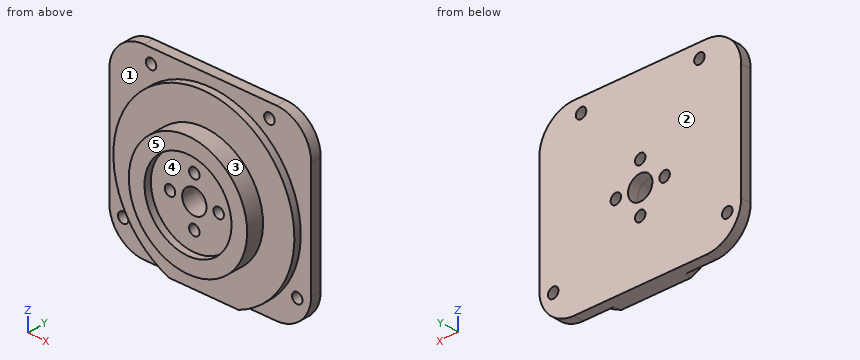
```python
from build123d import *
from build123d.topology import SkipClean

# Parameters (mm, degrees)
SKETCH_1_W          = 58
SKETCH_1_H          = 58
SKETCH_1_R          = 1.5
SKETCH_1_R_2        = 3.5
EXTRUDE_1_DEPTH     = 3
EXTRUDE_START       = 5
SKETCH_2_R          = 12.5
SKETCH_2_R_2        = 1.5
SKETCH_2_R_3        = 3.5
EXTRUDE_2_DEPTH     = 5
EXTRUDE_START_2     = 7
SKETCH_6_R          = 17
SKETCH_6_R_2        = 12.5
EXTRUDE_3_DEPTH     = 7
SKETCH_8_R          = 26
SKETCH_8_R_2        = 12
EXTRUDE_5_DEPTH     = 2
SKETCH_10_W         = 58
SKETCH_10_H         = 5
CUT_EXTRUDE_1_DEPTH = 10
FILLET_1_R          = 10


with BuildPart() as part:
    # 草图1 → 凸台-拉伸1 (new body)
    with BuildSketch(Plane(origin=(0, 0, 0), x_dir=(1, 0, 0), z_dir=(0, 1, 0))):
        Rectangle(SKETCH_1_W, SKETCH_1_H)
        with Locations(Location((0, 7, 0), (0, 0, 270))):
            Circle(SKETCH_1_R, mode=Mode.SUBTRACT)
        with Locations(Location((7, 0, 0), (0, 0, 270))):
            Circle(SKETCH_1_R, mode=Mode.SUBTRACT)
        with Locations(Location((0, 0, 0), (0, 0, 270))):
            Circle(SKETCH_1_R_2, mode=Mode.SUBTRACT)
        with Locations(Location((0, -7, 0), (0, 0, 90))):
            Circle(SKETCH_1_R, mode=Mode.SUBTRACT)
        with Locations(Location((-7, 0, 0), (0, 0, 90))):
            Circle(SKETCH_1_R, mode=Mode.SUBTRACT)
        with Locations(Location((25, 16, 0), (0, 0, 270))):
            Circle(SKETCH_1_R, mode=Mode.SUBTRACT)
        with Locations(Location((-25, 16, 0), (0, 0, 90))):
            Circle(SKETCH_1_R, mode=Mode.SUBTRACT)
        with Locations(Location((17, -25, 0), (0, 0, 270))):
            Circle(SKETCH_1_R, mode=Mode.SUBTRACT)
        with Locations(Location((-17, -25, 0), (0, 0, 90))):
            Circle(SKETCH_1_R, mode=Mode.SUBTRACT)
    extrude(amount=EXTRUDE_1_DEPTH)

    # 草图2 → 凸台-拉伸2 (add)
    with SkipClean():  # the faces are left unmerged after this step: merging them gives an invalid solid
        with BuildSketch(Plane.XZ.offset(EXTRUDE_START)):
            with Locations(Location((0, 0, 0), (0, 0, 270))):
                Circle(SKETCH_2_R)
            with Locations(Location((0, 7, 0), (0, 0, 270))):
                Circle(SKETCH_2_R_2, mode=Mode.SUBTRACT)
            with Locations(Location((0, 0, 0), (0, 0, 270))):
                Circle(SKETCH_2_R_3, mode=Mode.SUBTRACT)
            with Locations(Location((-7, 0, 0), (0, 0, 270))):
                Circle(SKETCH_2_R_2, mode=Mode.SUBTRACT)
            with Locations(Location((0, -7, 0), (0, 0, 270))):
                Circle(SKETCH_2_R_2, mode=Mode.SUBTRACT)
            with Locations(Location((7, 0, 0), (0, 0, 270))):
                Circle(SKETCH_2_R_2, mode=Mode.SUBTRACT)
        extrude(amount=-EXTRUDE_2_DEPTH)

    # 草图6 → 凸台-拉伸3 (add)
    with SkipClean():  # the faces are left unmerged after this step: merging them gives an invalid solid
        with BuildSketch(Plane.XZ.offset(EXTRUDE_START_2)):
            with Locations(Location((0, 0, 0), (0, 0, 270))):
                Circle(SKETCH_6_R)
            with Locations(Location((0, 0, 0), (0, 0, 270))):
                Circle(SKETCH_6_R_2, mode=Mode.SUBTRACT)
        extrude(amount=-EXTRUDE_3_DEPTH)

    # 草图8 → 凸台-拉伸5 (add)
    with SkipClean():  # the faces are left unmerged after this step: merging them gives an invalid solid
        with BuildSketch(Plane.XZ):
            with Locations(Location((0, 0, 0), (0, 0, 270))):
                Circle(SKETCH_8_R)
            Circle(SKETCH_8_R_2, mode=Mode.SUBTRACT)
        extrude(amount=EXTRUDE_5_DEPTH)

    # 草图10 → 切除-拉伸1 (cut)
    with BuildSketch(Plane(origin=(0, 3, 0), x_dir=(1, 0, 0), z_dir=(0, 1, 0))):
        with Locations((0, 26.5)):
            Rectangle(SKETCH_10_W, SKETCH_10_H)
    extrude(amount=-CUT_EXTRUDE_1_DEPTH, mode=Mode.SUBTRACT)

    # 圆角1
    fillet_1_edges = [part.edges().sort_by_distance(p)[0] for p in [
        (29, 1.5, 29),
        (-29, 1.5, 29),
        (29, 1.5, -24),
        (-29, 1.5, -24),
    ]]
    fillet(fillet_1_edges, radius=FILLET_1_R)


solid = part.part
```
For this review, take the finished solid that the model builds, in its own axes (mm). Face numbers are marked on the shaded views. A direction names the side the tool comes from. Give positions to 0.01 mm unless a question says otherwise; leave off trailing zeros. Write each loop counter-clockwise with the first axis right and the second up, starting at its lowest first coordinate (ties: lowest second). Pieces come first, ordered by that corner, then holes. Notation, with made-up numbers: M -3.75,26.5 L 3.25,26.5 A19 ccw 3.25,39.5 Z; hole C 71.25,14 d5. An arc over 180 degrees is marked long. Answer as a JSON object with one key per item and string values. Group by question number.
Item 1: Tool access review of the marked faces 1 and 2: name each direction out of +Z, -Z, +X, -X, +Y, -Y from which nothing blocks a thin tool from reaching the whole face with its end or side.
Item 2: For pin 1 Ø6 at (x, y) = (-21, 0) entering from -Z; pin 2 Ø1.8 at (x, z) = (17, 25) entering from +Y; pin 3 Ø8 at (x, z) = (-5, -1) entering from -Y; pin 4 Ø5 at (y, z) = (-3, -11) entering from +X, all flat-tipped, find the tip position at first contact; note any pin that passes through.
Item 3: Draft analysis for pull direction X (two halves, no side actions). For the marked faces 3, 4 and 5, state which applies: +X half, -X half, draft (parallel to the pull), parting line (faces both ways), or undercut.
Item 4: For probe 1 along X at (y, z) = (1.45, 0); probe 2 along Z at (x, y) = (0, 0.65); probe 3 along Z at (x, y) = (-17, 1.8), list the stretches that pass through material, from the lowest coordinate up. Write a range as [from, to].
Item 5: Consider section A-A on x = 0. Write out the cut boundary in (y, z).
Item 6: Consider section B-B on y = -3.75. Write out the cut boundary in (x, z), plus the area to 3 significant figures.
Item 7: Consider section D-D on z = -7. Write out the cut boundary in (x, y).
Item 8: Consider section C-C on x = 25. Write out the cut boundary in (y, z).
Check result:
{
 "1": {"face 1": "-Y", "face 2": "+Z, -Z, +X, -X, +Y"},
 "2": {"pin 1": "stops at z = -24", "pin 2": "passes through", "pin 3": "stops at y = -5", "pin 4": "stops at x = 24.5"},
 "3": {"face 3": "parting line", "face 4": "undercut", "face 5": "draft"},
 "4": {"probe 1": "x = [-29, -8.5], [-5.5, -3.5], [3.5, 5.5], [8.5, 29]", "probe 2": "z = [-24, -8.5], [-5.5, -3.5], [3.5, 5.5], [8.5, 29]", "probe 3": "z = [-24, 23.5], [26.5, 29]"},
 "5": {"outline": "M -7,-17 L -2,-17 L -2,-24 L 3,-24 L 3,-8.5 L -5,-8.5 L -5,-12.5 L -7,-12.5 Z; M -7,12.5 L -5,12.5 L -5,8.5 L 3,8.5 L 3,29 L 0,29 L 0,26 L -2,26 L -2,17 L -7,17 Z; M -5,-5.5 L 3,-5.5 L 3,-3.5 L -5,-3.5 Z; M -5,3.5 L 3,3.5 L 3,5.5 L -5,5.5 Z"},
 "6": {"outline": "C 0,0 d34; hole C -7,0 d3; hole C 0,0 d7; hole C 0,-7 d3; hole C 0,7 d3; hole C 7,0 d3", "area": "841 mm^2"},
 "7": {"outline": "M -29,0 L -25.04,0 L -25.04,-2 L -15.49,-2 L -15.49,-7 L -10.36,-7 L -10.36,-5 L -1.5,-5 L -1.5,3 L -29,3 Z; M 1.5,-5 L 10.36,-5 L 10.36,-7 L 15.49,-7 L 15.49,-2 L 25.04,-2 L 25.04,0 L 29,0 L 29,3 L 1.5,3 Z"},
 "8": {"outline": "M -2,-7.14 L 0,-7.14 L 0,-14.5 L 3,-14.5 L 3,27 L 0,27 L 0,7.14 L -2,7.14 Z; M 0,-22 L 3,-22 L 3,-17.5 L 0,-17.5 Z"}
}
